```python
from build123d import *

# Parameters (mm, degrees)
F0_R          = 50.0571816825
F1_DEPTH      = 500
F2_R          = 25.188754889
F3_DEPTH      = 170
F4_R          = 39.6850141268
F4_R_2        = 12.9457043272
F5_DEPTH      = 12.5
F6_R          = 12.6289029658
F7_DEPTH      = 50.0581816825
F7_DEPTH_BACK = 50.0581816825
F8_R          = 14.5825404329
F8_R_2        = 10.3798994513
F9_DEPTH      = 70
F10_R         = 15.1304262214
F10_R_2       = 10.1486644431
F11_DEPTH     = 70


with BuildPart() as f1:
    # F0 (on Front) → F1 (new body)
    with BuildSketch(Plane.XZ):
        Circle(F0_R)
    extrude(amount=F1_DEPTH)

    # F2 (on Front) → F3 (join)
    with BuildSketch(Plane.XZ):
        Circle(F2_R)
    extrude(amount=-F3_DEPTH)

    # F4 (on Right) → F5 (join, symmetric)
    with BuildSketch(Plane.YZ):
        with Locations((203.7855833769, 0)):
            Circle(F4_R)
        with Locations((203.7855833769, 0)):
            Circle(F4_R_2, mode=Mode.SUBTRACT)
    extrude(amount=F5_DEPTH, both=True)

    # F6 (on Right) → F7 (cut, two sides)
    with BuildSketch(Plane.YZ) as f7_sk:
        with Locations((-465.4365181923, 0)):
            Circle(F6_R)
    extrude(amount=-F7_DEPTH, mode=Mode.SUBTRACT)
    extrude(f7_sk.sketch, amount=F7_DEPTH_BACK, mode=Mode.SUBTRACT)

    # F8 (on Top) → F9 (join)
    with BuildSketch(Plane.XY):
        with Locations((0, -40.1445440948)):
            Circle(F8_R)
        with Locations((0, -40.1445440948)):
            Circle(F8_R_2, mode=Mode.SUBTRACT)
    extrude(amount=F9_DEPTH)

    # F10 (on Top) → F11 (join)
    with BuildSketch(Plane.XY):
        with Locations((0, -386.5570127964)):
            Circle(F10_R)
        with Locations((0, -386.5570127964)):
            Circle(F10_R_2, mode=Mode.SUBTRACT)
    extrude(amount=F11_DEPTH)


solid = f1.part
```
Build history of the part. All positions in model axes, mm. A direction names the side the tool comes from. Coordinates: 2 decimals unless noted, no trailing zeros. Order: outer loops, then holes, each group sorted by start corner. A loop starts at its lowest first (then second) coordinate and runs counter-clockwise, first axis right, second up. Notation, with made-up numbers: (54, 16) -> (84, 16) arc R25 ccw to (84, 52) -> close; hole circle Ø9 at (32.25, -31.5). An arc over 180 degrees is marked (long way). Answer in a Markdown table with one row per item. Add a question column.
Q1. Band-saw the part on C-C, the plane y = -363. List the corners of the cut face in (x, z).
Q2. Mould opens along Y. For faces 6 (the face through (-1, -500, 1)), 7 (the face through (6.98, -399.98, 58.7)), 8 (the face through (-12.5, 214.4, -8.3)) say: +Y half, -Y half, draft (parallel to the pull), parting line (faces both ways), or undercut.
Q3. Drop flat-ended pins along their axis: pin 1 (22 mm diameter, centred on y = 219, z = 10.5, fed in from +X); pin 2 (23.5 mm diameter, centred on x = 0, y = -386.56, fed in from -Z); pin 3 (23.5 mm diameter, centred on y = 203.79, z = 0, fed in from +X); pin 4 (3 mm diameter, centred on y = -190.5, z = -5.5, fed in from -X). Give the stop position or say it passes through.
Q4. Band-saw the part on B-B, the plane y = 41. List the corners of the cut face in (x, z).
Q5. Band-saw the part on A-A, the plane z = 0. List the corners of the cut face in (x, y), then the cut area to 3 significant figures.
Q6. Which spindle directions (+Z, -Z, +X, -X, +Y, -Y) get a long thin tool onto all of the face, cutting with end or side? Do faces 1 (the face through (-5.46, 83.81, -24.59)), 2 (the face through (12.5, 214.4, -8.3)), 3 (the face through (-0.175, 190.852, 0.569)), 4 (the face through (-2.2, -396.464, 59.362)), 5 (the face through (3.2, -396.4, 70)). Say none if no direction does.
Q7. Wall check: line 1 along Y through (x, z) = (0, 60.5); line 2 along Y through (x, z) = (27, 0); line 3 along Y through (x, z) = (-20, 0). Give the ranges that are in metal, low to high. Write a range as [from, to].
Answers follow:
| question | item | result |
|---|---|---|
| 1 | outline | circle Ø100.11 at (0, 0) |
| 2 | face 6 | -Y half |
| 2 | face 7 | undercut |
| 2 | face 8 | draft |
| 3 | pin 1 | x = 12.5 |
| 3 | pin 2 | z = -50.06 |
| 3 | pin 3 | through |
| 3 | pin 4 | x = -49.9 |
| 4 | outline | circle Ø50.38 at (0, 0) |
| 5 | outline | (-50.06, -500) -> (50.06, -500) -> (50.06, -478.07) -> (-50.06, -478.07) -> close; (-50.06, -452.81) -> (50.06, -452.81) -> (50.06, 0) -> (25.19, 0) -> (25.19, 170) -> (12.5, 170) -> (12.5, 190.84) -> (-12.5, 190.84) -> (-12.5, 170) -> (-25.19, 170) -> (-25.19, 0) -> (-50.06, 0) -> close; (-12.5, 216.73) -> (12.5, 216.73) -> (12.5, 243.47) -> (-12.5, 243.47) -> close |
| 5 | area | 57,300 mm^2 |
| 6 | face 1 | none |
| 6 | face 2 | +Z, -Z, +X, +Y |
| 6 | face 3 | +X, -X |
| 6 | face 4 | +Z |
| 6 | face 5 | +Z, +X, -X, +Y, -Y |
| 7 | line 1 | [-401.69, -396.71], [-376.41, -371.43], [-54.73, -50.52], [-29.76, -25.56] |
| 7 | line 2 | [-500, -478.07], [-452.81, 0] |
| 7 | line 3 | [-500, -478.07], [-452.81, 170] |
